The model under review builds one solid part; all positions refer to its coordinate system, in mm. A direction names the side the tool comes from. Round coordinates to 2 decimals unless told otherwise and drop trailing zeros. Order: outer loops, then holes, each group sorted by start corner. A loop starts at its lowest first (then second) coordinate and runs counter-clockwise, first axis right, second up. Notation, with made-up numbers: M 30.5,56 L 70.5,56 A14 cw 70.5,82 Z; hole C 20,-20.5 d5. An arc over 180 degrees is marked long. Answer as a JSON object with one key per item and string values. Group by question number.
1) Consider section D-D, the plane y = -6. Write out the cut boundary in (x, z).
2) For faces 5 (the flat face through (32.95, -25, 1)), 6 (the flat face through (-3, 25, 1.4)), 7 (the flat face through (-28, -17, 1.4)), 8 (the flat face through (32.95, 20, 1)), list the 3-axis set-ups (+Z, -Z, +X, -X, +Y, -Y) from which the entire face can be reached by the end or side of a thin tool; tool diameter is ignored.
3) Insertion check: pin 1 Ø4 at (x, y) = (-30.5, 12) entering from +Z; pin 2 Ø7 at (x, y) = (-8.55, -16.75) entering from +Z. Each pin has a flat end and moves straight along its axis. Give the tip position at first contact, or say it passes through.
4) Consider section C-C, the plane x = 23. Write out the cut boundary in (y, z).
5) To check wall thickness, follow line 1 (Y direction, x = -16.55, z = 1.45); line 2 (Y direction, x = -26.5, z = 1.45); line 3 (X direction, y = -24.25, z = 0.6). State the ranges of each line that lie inside material, in increasing order.
6) Consider section A-A, the plane y = 24.25. Write out the cut boundary in (x, z), then the cut area to 3 significant figures.
7) The part is to be moulded in two halves that separate along Y. For faces 1 (the flat face through (-29, 11, 1.4)), 2 (the flat face through (-17, -17, 1.4)), 3 (the flat face through (0, 26.75, 1)), 4 (the flat face through (2, 0, 1.5)), say which applies: +Y half, -Y half, draft (parallel to the pull), parting line (faces both ways), or undercut.
8) Consider section B-B, the plane z = 0.4. Write out the cut boundary in (x, y), then the cut area to 3 significant figures.
```python
from build123d import *

# Parameters (mm, degrees)
ESQUISSE1_R             = 1.5
BOSS_EXTRU_1_DEPTH      = 1.5
ESQUISSE2_R             = 3
ESQUISSE2_W             = 6.5
ESQUISSE2_H             = 6.5
ESQUISSE2_W_2           = 36
ESQUISSE2_H_2           = 10
ESQUISSE2_W_3           = 5
ESQUISSE2_H_3           = 7.5
ESQUISSE2_W_4           = 20
ESQUISSE2_H_4           = 2.3
ESQUISSE2_W_5           = 15
ESQUISSE2_W_6           = 10.797288279
ESQUISSE2_H_5           = 8.8
ESQUISSE2_W_7           = 11.916291933
ESQUISSE2_H_6           = 12
ESQUISSE2_W_8           = 25
ESQUISSE2_W_9           = 7.5
ESQUISSE2_H_7           = 5
ENL_V_MAT_EXTRU_1_DEPTH = 0.1


with BuildPart() as part:
    # Esquisse1 → Boss.-Extru.1 (new body)
    with BuildSketch(Plane.XY):
        Polygon((35.75, 10.45), (35.75, -21.75), (32.95, -23.75), (32.95, -26.75), (-32.95, -26.75), (-32.95, 26.75), (32.95, 26.75), (32.95, 13.25), align=None)
        with Locations((33.25, 9.25)):
            Circle(ESQUISSE1_R, mode=Mode.SUBTRACT)
        with Locations((33.25, -18.75)):
            Circle(ESQUISSE1_R, mode=Mode.SUBTRACT)
        with Locations((-19.45, 24.25)):
            Circle(ESQUISSE1_R, mode=Mode.SUBTRACT)
        with Locations(Location((-19.45, -24.25, 0), (0, 0, 180))):
            Circle(ESQUISSE1_R, mode=Mode.SUBTRACT)
    extrude(amount=BOSS_EXTRU_1_DEPTH)

    # Esquisse2 → Enlèv. mat.-Extru.1 (cut)
    with BuildSketch(Plane.XY.offset(1.5)):
        with Locations((-16.55, -16.75)):
            Circle(ESQUISSE2_R)
        with Locations((-8.55, -16.75)):
            Circle(ESQUISSE2_R)
        with Locations((-26.7, 22.5)):
            Rectangle(ESQUISSE2_W, ESQUISSE2_H)
        with BuildLine():
            Line((-18.45, 0.25), (-11.45, 0.25))
            ThreePointArc((-11.45, 0.25), (-9.95, -1.25), (-11.45, -2.75))
            Line((-11.45, -2.75), (-18.45, -2.75))
            ThreePointArc((-18.45, -2.75), (-19.95, -1.25), (-18.45, 0.25))
        make_face()
        with Locations((12.75, -9.75)):
            Rectangle(ESQUISSE2_W_2, ESQUISSE2_H_2)
        with Locations((32.25, 1)):
            Rectangle(ESQUISSE2_W_3, ESQUISSE2_H_3)
        with Locations((4.05, -24.6)):
            Rectangle(ESQUISSE2_W_4, ESQUISSE2_H_4)
        with Locations((24.45, -24.6)):
            Rectangle(ESQUISSE2_W_5, ESQUISSE2_H_4)
        with Locations((-28.34864414, -17.35)):
            Rectangle(ESQUISSE2_W_6, ESQUISSE2_H_5)
        with Locations((-30.908145967, 10.75)):
            Rectangle(ESQUISSE2_W_7, ESQUISSE2_H_6)
        with Locations((-2.45, 24.6)):
            Rectangle(ESQUISSE2_W_8, ESQUISSE2_H_4)
        with Locations((21.95, 24.6)):
            Rectangle(ESQUISSE2_W_4, ESQUISSE2_H_4)
        with Locations((-13.2, 19.25)):
            Rectangle(ESQUISSE2_W_9, ESQUISSE2_H_7)
    extrude(amount=-ENL_V_MAT_EXTRU_1_DEPTH, mode=Mode.SUBTRACT)


solid = part.part
```
Results list:
{
 "1": {"outline": "M -32.95,0 L 35.75,0 L 35.75,1.5 L 30.75,1.5 L 30.75,1.4 L -5.25,1.4 L -5.25,1.5 L -32.95,1.5 Z"},
 "2": {"face 5": "+Z, -Z, +X, -Y", "face 6": "+Z", "face 7": "+Z, -X", "face 8": "+Z, -Z, +X, +Y"},
 "3": {"pin 1": "z = 1.4", "pin 2": "z = 1.5"},
 "4": {"outline": "M -26.75,0 L 26.75,0 L 26.75,1.5 L 25.75,1.5 L 25.75,1.4 L 23.45,1.4 L 23.45,1.5 L -4.75,1.5 L -4.75,1.4 L -14.75,1.4 L -14.75,1.5 L -23.45,1.5 L -23.45,1.4 L -25.75,1.4 L -25.75,1.5 L -26.75,1.5 Z"},
 "5": {"line 1": "-26.75 to -19.75, -13.75 to -2.75, 0.25 to 16.75, 21.75 to 26.75", "line 2": "-26.75 to -21.75, -12.95 to 4.75, 16.75 to 19.25, 25.75 to 26.75", "line 3": "-32.95 to -20.95, -17.95 to 32.95"},
 "6": {"outline": "M -32.95,0 L -20.95,0 L -20.95,1.5 L -23.45,1.5 L -23.45,1.4 L -29.95,1.4 L -29.95,1.5 L -32.95,1.5 Z; M -17.95,0 L 32.95,0 L 32.95,1.5 L 31.95,1.5 L 31.95,1.4 L 11.95,1.4 L 11.95,1.5 L 10.05,1.5 L 10.05,1.4 L -14.95,1.4 L -14.95,1.5 L -17.95,1.5 Z", "area": "89.2 mm^2"},
 "7": {"face 1": "undercut", "face 2": "undercut", "face 3": "+Y half", "face 4": "draft"},
 "8": {"outline": "M -32.95,-26.75 L 32.95,-26.75 L 32.95,-23.75 L 35.75,-21.75 L 35.75,10.45 L 32.95,13.25 L 32.95,26.75 L -32.95,26.75 Z; hole C -19.45,-24.25 d3; hole C -19.45,24.25 d3; hole C 33.25,-18.75 d3; hole C 33.25,9.25 d3", "area": "3,590 mm^2"}
}
